```python
from build123d import *

# Parameters (mm, degrees)
F0_W      = 65
F0_H      = 126
F1_DEPTH  = 12
F2_R      = 16
F3_R      = 8
F4_DEPTH  = 12
F5_R      = 26
F6_DEPTH  = 34
F7_R      = 30
F8_DEPTH  = 12
F9_R      = 15
F10_DEPTH = 12
F11_R     = 10
F12_DEPTH = 46
F14_DEPTH = 46
F15_W     = 8
F15_H     = 43
F16_DEPTH = 46
F18_DEPTH = 8


with BuildPart() as f1:
    # F0 (on Top) → F1 (new body)
    with BuildSketch(Plane.XY):
        Rectangle(F0_W, F0_H)
    extrude(amount=F1_DEPTH)

    # F2
    f2_edges = [f1.edges().sort_by_distance(p)[0] for p in [
        (32.5, -63, 6),
        (-32.5, -63, 6),
        (32.5, 63, 6),
        (-32.5, 63, 6),
    ]]
    fillet(f2_edges, radius=F2_R)

    # F3 (on face) → F4 (cut, through all)
    with BuildSketch(Plane.XY.offset(12)):
        with Locations((-16.5, 48)):
            Circle(F3_R)
        with Locations((16.5, 48)):
            Circle(F3_R)
        with Locations((16.5, -48)):
            Circle(F3_R)
        with Locations((-16.5, -48)):
            Circle(F3_R)
    extrude(amount=-F4_DEPTH, mode=Mode.SUBTRACT)

    # F5 (on face) → F6 (join)
    with BuildSketch(Plane.XY.offset(12)):
        Circle(F5_R)
    extrude(amount=F6_DEPTH)

    # F7 (on face) → F8 (join)
    with BuildSketch(Plane.XY.offset(46)):
        Circle(F7_R)
    extrude(amount=F8_DEPTH)

    # F9 (on face) → F10 (cut)
    with BuildSketch(Plane.XY.offset(58)):
        Circle(F9_R)
    extrude(amount=-F10_DEPTH, mode=Mode.SUBTRACT)

    # F11 (on face) → F12 (cut, through all)
    with BuildSketch(Plane.XY.offset(46)):
        Circle(F11_R)
    extrude(amount=-F12_DEPTH, mode=Mode.SUBTRACT)

    # F13 (on face) → F14 (cut, through all)
    with BuildSketch(Plane.XY.offset(58)):
        with BuildLine():
            Line((22.36068, -20), (-22.36068, -20))
            ThreePointArc((-22.36068, -20), (0, -30), (22.36068, -20))
        make_face()
    extrude(amount=-F14_DEPTH, mode=Mode.SUBTRACT)

    # F15 (on face) → F16 (join, through all)
    with BuildSketch(Plane.XY.offset(12)):
        with Locations((0, -41.5)):
            Rectangle(F15_W, F15_H)
    extrude(amount=F16_DEPTH)

    # F17 (on face) → F18 (cut, through all)
    with BuildSketch(Plane.YZ.offset(4)):
        Polygon((-63, 12), (-20, 58), (-63, 58), align=None)
    extrude(amount=-F18_DEPTH, mode=Mode.SUBTRACT)


solid = f1.part
```
Design review of the part built by this model. Coordinates are the model's own, in mm. A direction names the side the tool comes from. Coordinates: 2 decimals unless noted, no trailing zeros. Write each loop counter-clockwise with the first axis right and the second up, starting at its lowest first coordinate (ties: lowest second). Pieces come first, ordered by that corner, then holes.
1) Add section A-A (y = 0). Write out the cut boundary in (x, z).
2) Add section C-C (z = 51). Write out the cut boundary in (x, y).
3) Machinability: for faces 4 (the flat face through (0, -13, 0)), 5 (the cylindrical face through (0.891, 25.985, 28.762)), 6 (the flat face through (3, -10, 46)), 7 (the flat face through (11, -20, 35)), which of the approach directions +Z, -Z, +X, -X, +Y, -Y give a long, thin tool a straight path to every point of the face, cutting with its end or side? Answer none if there is none.
4) Mouldability with a two-part tool opening along Y and no side actions: class faces 1 (the cylindrical face through (-17.541, -40.068, 6.084)), 2 (the flat face through (-4, -32, 24)), 3 (the cylindrical face through (0.966, 29.984, 51.916)) as +Y half, -Y half, draft (parallel to the pull), parting line (faces both ways), or undercut.
5) Add section D-D (x = 13.5). Write out the cut boundary in (y, z).
6) To check wall thickness, follow L1, parallel to Y at x = 16, z = 6; L2, parallel to Z at x = -8.5, y = 28.5; L3, parallel to Z at x = -22, y = 40.5. State the ranges of each line that lie inside material, in increasing order.
7) Insertion check: pin 1 (6 mm diameter, centred on y = 11, z = 41, fed in from +X); pin 2 (18.5 mm diameter, centred on x = -16.5, y = -48, fed in from +Z); pin 3 (14.5 mm diameter, centred on x = -17, z = 45, fed in from -Y). Each pin has a flat end and moves straight along its axis. Give the tip position at first contact, or say it passes through.
8) Add section B-B (x = 0). Write out the cut boundary in (y, z).
Check result:
1. outline: (-32.5, 0) - (-10, 0) - (-10, 46) - (-15, 46) - (-15, 58) - (-30, 58) - (-30, 46) - (-26, 46) - (-26, 12) - (-32.5, 12) - close; (10, 0) - (32.5, 0) - (32.5, 12) - (26, 12) - (26, 46) - (30, 46) - (30, 58) - (15, 58) - (15, 46) - (10, 46) - close
2. outline: (-22.36, -20) - (-4, -20) - (-4, -26.54) - (4, -26.54) - (4, -20) - (22.36, -20) arc R30 ccw (long way) to start; hole circle Ø30 at (0, 0)
3. face 4: -Z, +X, -X, +Y, -Y
3. face 5: none
3. face 6: +Z
3. face 7: +Z, +X, -Y
4. face 1: undercut
4. face 2: draft
4. face 3: parting line
5. outline: (-63, 0) - (-55.42, 0) - (-55.42, 12) - (-63, 12) - close; (-40.58, 0) - (40.58, 0) - (40.58, 12) - (22.22, 12) - (22.22, 46) - (26.79, 46) - (26.79, 58) - (6.54, 58) - (6.54, 46) - (-6.54, 46) - (-6.54, 58) - (-20, 58) - (-20, 12) - (-40.58, 12) - close; (55.42, 0) - (63, 0) - (63, 12) - (55.42, 12) - close
6. L1: y = -63 to -55.98, -40.02 to 40.02, 55.98 to 63
6. L2: z = 0 to 12, 46 to 58
6. L3: z = 0 to 12
7. pin 1: stops at x = 24.74
7. pin 2: stops at z = 12
7. pin 3: stops at y = -20
8. outline: (-63, 0) - (-10, 0) - (-10, 46) - (-15, 46) - (-15, 58) - (-20, 58) - (-63, 12) - close; (10, 0) - (63, 0) - (63, 12) - (26, 12) - (26, 46) - (30, 46) - (30, 58) - (15, 58) - (15, 46) - (10, 46) - close
